Verification items for the finished model (mm, model axes). A direction names the side the tool comes from. Give positions to 0.01 mm unless a question says otherwise; leave off trailing zeros. Loops run counter-clockwise (first coordinate to the right, second up) from the corner with the lowest first, then second, coordinate; pieces in that order, holes last. Notation, with made-up numbers: (46.25, -17) - (50.25, -17) arc R22 ccw to (50.25, 20) - close; hole circle Ø3 at (68.25, 79). An arc over 180 degrees is marked (long way). One line per item, written item: value. Start each with the question number.
1. Sectioned sample at A-A (y = -74). Record the cut outline in (x, z).
2. Mould release check, pull along X, two halves, no side actions. Record for faces 3 (the flat face through (-66, -41, 5)), 4 (the flat face through (-79.003, -59.809, 2.465)), 5 (the flat face through (-122.6, -65, 2.5)), 6 (the cylindrical face through (-1.32, 0.06, 2.46)): pulls with the +X half, pulls with the -X half, needs draft (parallel to the pull), parting line crosses it, or undercut.
3. Scan lines: L1, parallel to X at y = -30, z = 3.8; L2, parallel to Y at x = -99.5, z = 3.75; L3, parallel to X at y = -58.5, z = 0.6. Record each from-to range of solid material in increasing order. Write a range as [from, to].
4. Access from +Z, -Z, +X, -X, +Y, -Y to the whole of each face (thin tool, end or side, straight path). Record for faces 1 (the flat face through (-114.3, -70.866, 2.465)), 2 (the cylindrical face through (-51.24, -27.69, 2.46)).
5. Gauge pin test, flat ends, axial feed: pin 1 (3.5 mm diameter, centred on x = 0.28, y = -0.01, fed in from -Z); pin 2 (2 mm diameter, centred on y = -40, z = 1, fed in from +X); pin 3 (3 mm diameter, centred on y = -72, z = 1.5, fed in from +X); pin 4 (3 mm diameter, centred on y = -22.5, z = 1, fed in from +X). Record the tip position at first contact, or that the pin passes through.
6. Sectioned sample at C-C (x = -111). Record the cut outline in (y, z).
7. Sectioned sample at D-D (y = -10.5). Record the cut outline in (x, z), plus the area to 3 significant figures.
8. Sectioned sample at B-B (z = 3.2). Count the separate pieces of the cut face and the enclosed holes in it, plus the area to 3 significant figures.
from build123d import *

# Parameters (mm, degrees)
SKETCH1_R           = 3.5
SKETCH1_R_2         = 1.55
SKETCH1_R_3         = 1.6
BOSS_EXTRUDE1_DEPTH = 5


with BuildPart() as part:
    # Sketch1 → Boss-Extrude1 (new body)
    # profile 1 of 4: a face of its own
    with BuildSketch(Plane.XY):
        with BuildLine():
            ThreePointArc((-50.379412597, -32.059346711), (-54.886807697, -31.081444916), (-54.511132434, -26.484514353))
            Line((-54.511132434, -26.484514353), (-107.325001283, -77.686959994))
            Line((-107.325001283, -77.686959994), (-121.473901164, -63.850866788))
            Line((-121.473901164, -63.850866788), (-123.810410836, -66.240200318))
            Line((-123.810410836, -66.240200318), (-125.631536255, -68.068297032))
            Line((-125.631536255, -68.068297032), (-106.835385186, -86.792770537))
            Line((-106.835385186, -86.792770537), (-50.379412597, -32.059346711))
        make_face()
    # profile 2 of 4: a face of its own
    with BuildSketch(Plane.XY):
        with BuildLine():
            Line((-1.415959287, 3.054745501), (-53.770371078, -25.935507998))
            ThreePointArc((-53.770371078, -25.935507998), (-50.297840536, -25.982118304), (-48.574891838, -28.997427354))
            ThreePointArc((-48.574891838, -28.997427354), (-49.059582787, -30.774478656), (-50.379412597, -32.059346711))
            Line((-50.379412597, -32.059346711), (1.974999193, -3.069093212))
            ThreePointArc((1.974999193, -3.069093212), (-2.782399403, -1.702653096), (-1.415959287, 3.054745501))
        make_face()
    # profile 3 of 4: a face of its own
    with BuildSketch(Plane.XY):
        with Locations((-52.074891838, -28.997427354)):
            Circle(SKETCH1_R)
        with Locations((-52.074891838, -28.997427354)):
            Circle(SKETCH1_R_2, mode=Mode.SUBTRACT)
    # profile 4 of 4: a face of its own
    with BuildSketch(Plane.XY):
        with Locations((0.279519953, -0.007173855)):
            Circle(SKETCH1_R)
        with Locations((0.279519953, -0.007173855)):
            Circle(SKETCH1_R_3, mode=Mode.SUBTRACT)
    extrude(amount=BOSS_EXTRUDE1_DEPTH)


solid = part.part
Results are:
1. outline: (-119.68, 0) - (-111.1, 0) - (-111.1, 5) - (-119.68, 5) - close; (-103.52, 0) - (-93.64, 0) - (-93.64, 5) - (-103.52, 5) - close
2. face 3: needs draft
2. face 4: pulls with the +X half
2. face 5: pulls with the -X half
2. face 6: undercut
3. L1: x = [-58.14, -53.26], [-50.89, -46.66]
3. L2: y = [-79.68, -70.1]
3. L3: x = [-87.53, -77.65]
4. face 1: +Z, -Z, +Y
4. face 2: +Z, -Z
5. pin 1: stops at z = 0
5. pin 2: stops at x = -57.54
5. pin 3: stops at x = -90.03
5. pin 4: stops at x = -30.41
6. outline: (-82.64, 0) - (-74.09, 0) - (-74.09, 5) - (-82.64, 5) - close
7. outline: (-25.89, 0) - (-11.44, 0) - (-11.44, 5) - (-25.89, 5) - close
7. area: 72.3 mm^2
8. separate pieces: 1
8. enclosed holes: 2
8. area: 1,090 mm^2
